```python
from build123d import *

# Parameters (mm, degrees)
SKETCH1_R           = 15.24
SKETCH1_R_2         = 9.525
BOSS_EXTRUDE2_DEPTH = 12.7
SKETCH3_R           = 15.24
BOSS_EXTRUDE3_DEPTH = 12.7
SKETCH4_R           = 15.24
SKETCH4_R_2         = 6.096
BOSS_EXTRUDE4_DEPTH = 12.7
SKETCH5_W           = 2.032
SKETCH5_H           = 12.7
BOSS_EXTRUDE5_DEPTH = 12.7
BOSS_EXTRUDE6_START = -5.08
BOSS_EXTRUDE6_DEPTH = 5.08
SKETCH7_R           = 2.54
CUT_EXTRUDE1_DEPTH  = 5.08


with BuildPart() as part:
    # Sketch1 → Boss-Extrude2 (new body)
    with BuildSketch(Plane(origin=(0, 0, 0), x_dir=(1, 0, 0), z_dir=(0, 1, 0))):
        with Locations(Location((0, 0, 0), (0, 0, 270))):
            Circle(SKETCH1_R)
        with Locations(Location((0, 0, 0), (0, 0, 270))):
            Circle(SKETCH1_R_2, mode=Mode.SUBTRACT)
    extrude(amount=BOSS_EXTRUDE2_DEPTH)

    # Sketch3 → Boss-Extrude3 (add)
    with BuildSketch(Plane(origin=(0, 12.7, 0), x_dir=(1, 0, 0), z_dir=(0, 1, 0))):
        with Locations(Location((0, 0, 0), (0, 0, 270))):
            Circle(SKETCH3_R)
    extrude(amount=BOSS_EXTRUDE3_DEPTH)

    # Sketch4 → Boss-Extrude4 (add)
    with BuildSketch(Plane(origin=(0, 25.4, 0), x_dir=(1, 0, 0), z_dir=(0, 1, 0))):
        with Locations(Location((0, 0, 0), (0, 0, 270))):
            Circle(SKETCH4_R)
        with Locations(Location((0, 0, 0), (0, 0, 270))):
            Circle(SKETCH4_R_2, mode=Mode.SUBTRACT)
    extrude(amount=BOSS_EXTRUDE4_DEPTH)

    # Sketch5 → Boss-Extrude5 (add)
    with BuildSketch(Plane.XZ.offset(-12.7)):
        Rectangle(SKETCH5_W, SKETCH5_H)
    extrude(amount=BOSS_EXTRUDE5_DEPTH)

    # Sketch6 → Boss-Extrude6 (add)
    with BuildSketch(Plane(origin=(0, 38.1, 0), x_dir=(1, 0, 0), z_dir=(0, 1, 0)).offset(BOSS_EXTRUDE6_START)):
        with BuildLine():
            Line((-13.198227154, 7.62), (-33.02, 7.62))
            Line((-33.02, 7.62), (-33.02, -7.62))
            Line((-33.02, -7.62), (-13.198227154, -7.62))
            ThreePointArc((-13.198227154, -7.62), (-15.24, 0), (-13.198227154, 7.62))
        make_face()
    extrude(amount=BOSS_EXTRUDE6_DEPTH)

    # Sketch7 → Cut-Extrude1 (cut)
    with BuildSketch(Plane(origin=(0, 38.1, 0), x_dir=(1, 0, 0), z_dir=(0, 1, 0))):
        with Locations(Location((-25.4, 0, 0), (0, 0, 270))):
            Circle(SKETCH7_R)
    extrude(amount=-CUT_EXTRUDE1_DEPTH, mode=Mode.SUBTRACT)


solid = part.part
```
The model under review builds one solid part; all positions refer to its coordinate system, in mm. A direction names the side the tool comes from. Round coordinates to 2 decimals unless told otherwise and drop trailing zeros. Loops run counter-clockwise (first coordinate to the right, second up) from the corner with the lowest first, then second, coordinate; pieces in that order, holes last. Notation, with made-up numbers: M 41.5,39.25 L 51.5,39.25 A5 ccw 51.5,44.25 Z; hole C 28.25,-16 d2. An arc over 180 degrees is marked long. Put each result on its own line as item: value.
Q1. Consider section D-D, the plane x = 0. Give the boundary of the cut face in (y, z) (3 decimals), then the cut area to 3 significant figures.
Result set:
outline: M 0,-15.24 L 38.1,-15.24 L 38.1,-6.096 L 25.4,-6.096 L 25.4,6.096 L 38.1,6.096 L 38.1,15.24 L 0,15.24 L 0,9.525 L 12.7,9.525 L 12.7,6.35 L 0,6.35 L 0,-6.35 L 12.7,-6.35 L 12.7,-9.525 L 0,-9.525 Z
area: 926 mm²
Q2. Mouldability with a two-part tool opening along Z and no side actions: class faces 4 (the flat face through (0, 6, 6.35)), 5 (the flat face through (-23, 36, -7.62)), 6 (the flat face through (-23, 36, 7.62)) as released by +Z, released by -Z, zero draft, split by the parting line, or undercut.
Result set:
face 4: undercut
face 5: released by -Z
face 6: released by +Z
Q3. To check wall thickness, follow L1, parallel to X at y = 9, z = 0 (3 decimals); L2, parallel to X at y = 36.85, z = 0; L3, parallel to Z at x = -25, y = 36. State the ranges of each line that lie inside material, in increasing order.
Result set:
L1: x = -15.24 to -9.525, -1.016 to 1.016, 9.525 to 15.24
L2: x = -33.02 to -27.94, -22.86 to -6.1, 6.1 to 15.24
L3: z = -7.62 to -2.51, 2.51 to 7.62
Q4. Consider section C-C, the plane x = -25.4. Give the boundary of the cut face in (y, z), then the cut area to 3 significant figures.
Result set:
outline: M 33.02,-7.62 L 38.1,-7.62 L 38.1,-2.54 L 33.02,-2.54 Z; M 33.02,2.54 L 38.1,2.54 L 38.1,7.62 L 33.02,7.62 Z
area: 51.6 mm²
Q5. Consider section A-A, the plane y = 10.5. Give the boundary of the cut face in (x, z) (3 decimals), then the cut area to 3 significant figures.
Result set:
outline: C 0,0 d30.48; M -1.016,-6.35 L 1.016,-6.35 L 1.016,6.35 L -1.016,6.35 Z; hole C 0,0 d19.05
area: 470 mm²
Q6. Machinability: for faces 1 (the cylindrical face through (-5.796, 6.261, -7.559)), 2 (the flat face through (0, 25.4, 0)), 3 (the flat face through (-33.02, 36, 0)), which of the approach directions +Z, -Z, +X, -X, +Y, -Y give a long, thin tool a straight path to every point of the face, cutting with its end or side? Answer none if there is none.
Result set:
face 1: -Y
face 2: +Y
face 3: +Z, -Z, -X, +Y, -Y
Q7. For pin 1 (1 mm diameter, centred on y = 31, z = -3.5, fed in from -X); pin 2 (10 mm diameter, centred on x = -2, z = 4, fed in from +Y); pin 3 (5 mm diameter, centred on y = 4, z = -11, fed in from +X); pin 4 (4 mm diameter, centred on x = -20, y = 35, fed in from +Z), all flat-tipped, find the tip position at first contact; note any pin that passes through.
Result set:
pin 1: stops at x = -14.94
pin 2: stops at y = 38.1
pin 3: stops at x = 12.65
pin 4: stops at z = 7.62
Q8. Consider section B-B, the plane z = 0. Give the boundary of the cut face in (x, y) (3 decimals).
Result set:
outline: M -33.02,33.02 L -27.94,33.02 L -27.94,38.1 L -33.02,38.1 Z; M -22.86,33.02 L -15.24,33.02 L -15.24,0 L -9.525,0 L -9.525,12.7 L -1.016,12.7 L -1.016,0 L 1.016,0 L 1.016,12.7 L 9.525,12.7 L 9.525,0 L 15.24,0 L 15.24,38.1 L 6.096,38.1 L 6.096,25.4 L -6.096,25.4 L -6.096,38.1 L -22.86,38.1 Z
